Can you work these out from the model? Positions are in its coordinate system, mm. Face numbers are marked on the shaded views. A direction names the side the tool comes from. Round coordinates to 2 decimals unless told otherwise and drop trailing zeros. Order: outer loops, then holes, each group sorted by start corner. A loop starts at its lowest first (then second) coordinate and runs counter-clockwise, first axis right, second up. Notation, with made-up numbers: (49, 84) -> (62, 84) arc R14 ccw to (62, 106) -> close; hole circle Ø11 at (2.5, 27.5). An arc over 180 degrees is marked (long way). Use a Markdown table: item, result. Add a question column.
Q1. I'm going to push flat-ended pins straight in: pin 1 Ø1.4 at (x, z) = (3, 0.5) entering from -Y; pin 2 Ø2.5 at (x, z) = (8, 0.5) entering from -Y. Where does each tip first touch, or does it pass through?
Q2. If we section it at C-C on z = -2.25: List the corners of the cut face in (x, y) for me, plus the area to 3 significant figures.
Q3. If we section it at D-D on y = 6: List the corners of the cut face in (x, z) for me, plus the area to 3 significant figures.
Q4. For the marked faces 1, 2 and 3, which set-ups out of +Z, -Z, +X, -X, +Y, -Y let a thin tool reach every point of the face, with its end or its side?
Q5. We'd pull the mould along X, two halves only. Please class the marked faces 4, 5 and 6: +X half, -X half, draft (parallel to the pull), parting line (faces both ways), or undercut.
Q6. If we section it at B-B on y = 14.5: List the corners of the cut face in (x, z) for me, plus the area to 3 significant figures.
Q7. I need wall thicknesses on line 1 along Z through (x, y) = (3, 3.25); line 2 along Z through (x, y) = (5.5, 12.5); line 3 along X through (y, z) = (14.5, 0). Which ranges of each line are inside material? Lowest first, please. Write a range as [from, to].
Q8. If we section it at A-A on z = 0: List the corners of the cut face in (x, y) for me.
```python
from build123d import *

# Parameters (mm, degrees)
BOSS_EXTRUDE1_DEPTH      = 4
BOSS_EXTRUDE1_DEPTH_BACK = 4
SKETCH1_W                = 9.25
SKETCH1_H                = 17
CUT_EXTRUDE1_DEPTH       = 1.9
CUT_EXTRUDE1_DEPTH_BACK  = 1.9
SKETCH2_W                = 9.25
SKETCH2_H                = 12
SKETCH3_R                = 2.54
CUT_EXTRUDE2_DEPTH       = 21.941883869
FILLET1_R                = 0.5
CUT_EXTRUDE5_DEPTH       = 21.941884033
CUT_EXTRUDE6_REACH       = 20.488
SKETCH9_W                = 1.000000032
SKETCH9_H                = 8


# Read off the part's stored shape, not the designer's step: #10-32 Tapped Hole1
with BuildPart() as part:
    # Sketch1 → Boss-Extrude1 (new, two sides: drawn at the far end of the back side and taken through both)
    with BuildSketch(Plane.XY.offset(-BOSS_EXTRUDE1_DEPTH_BACK)):
        with Locations((4.625, 8.5)):
            Rectangle(SKETCH1_W, SKETCH1_H)
    extrude(amount=BOSS_EXTRUDE1_DEPTH + BOSS_EXTRUDE1_DEPTH_BACK)

    # Sketch2 → Cut-Extrude1 (cut, two sides: drawn at the far end of the back side and taken through both)
    with BuildSketch(Plane.XY.offset(-CUT_EXTRUDE1_DEPTH_BACK)):
        with Locations((4.625, 6)):
            Rectangle(SKETCH2_W, SKETCH2_H)
    extrude(amount=CUT_EXTRUDE1_DEPTH + CUT_EXTRUDE1_DEPTH_BACK, mode=Mode.SUBTRACT)

    # Sketch3 → Cut-Extrude2 (cut, through all)
    with BuildSketch(Plane.XY.offset(4)):
        with Locations((5.25, 5.5)):
            Circle(SKETCH3_R)
    extrude(amount=-CUT_EXTRUDE2_DEPTH, mode=Mode.SUBTRACT)

    # #10-32 Tapped Hole1 outline → #10-32 Tapped Hole1 (revolve, cut)
    with BuildSketch(Plane(origin=(5.5, 0, 0), x_dir=(1, 0, 0), z_dir=(0, 0, 1))):
        Polygon((0, 7.973018958), (1.928351252, 7.973018958), (2.019302964, 8.027668689), (2.0193, 17), (0, 17), align=None)
    revolve(axis=Axis((5.5, 0, 0), (0, 1, 0)), mode=Mode.SUBTRACT)

    # Fillet1
    fillet1_edges = [part.edges().sort_by_distance(p)[0] for p in [
        (7.716900739, 12, -1.9),
        (7.716900739, 12, 1.9),
        (2.408099261, 12, -1.9),
        (2.408099261, 12, 1.9),
    ]]
    fillet(fillet1_edges, radius=FILLET1_R)

    # Sketch7 → Cut-Extrude5 (cut, through all)
    with BuildSketch(Plane.XY.offset(4)):
        with BuildLine():
            Line((5.25, 1.5), (0, 1.5))
            Line((0, 1.5), (0, 0))
            Line((0, 0), (9.25, 0))
            Line((9.25, 0), (9.25, 5.5))
            ThreePointArc((9.25, 5.5), (8.078427125, 2.671572875), (5.25, 1.5))
        make_face()
    extrude(amount=-CUT_EXTRUDE5_DEPTH, mode=Mode.SUBTRACT)

    # Sketch9 → Cut-Extrude6 (cut, up to next)
    with BuildSketch(Plane(origin=(0, 17, 0), x_dir=(1, 0, 0), z_dir=(0, 1, 0)), mode=Mode.PRIVATE) as cut_extrude6_sk1:
        with Locations((0.500000016, 0)):
            Rectangle(SKETCH9_W, SKETCH9_H)
    cut_extrude6_tool1 = extrude(cut_extrude6_sk1.sketch, amount=-CUT_EXTRUDE6_REACH, mode=Mode.PRIVATE) & part.part
    add(cut_extrude6_tool1.solids().sort_by_distance((0.5, 17, 0))[0], mode=Mode.SUBTRACT)


solid = part.part
```
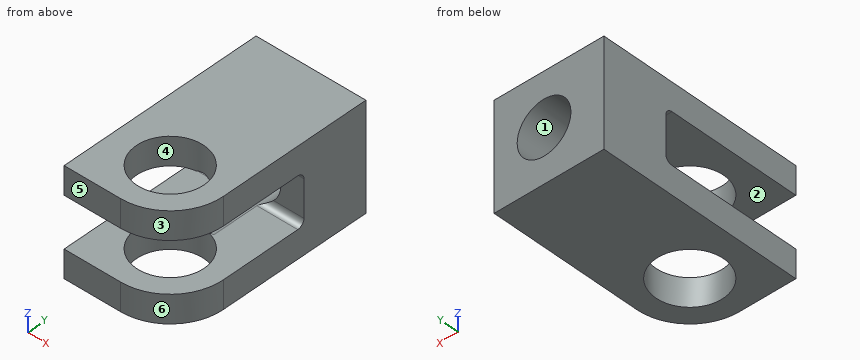
Answer below:
| question | item | result |
|---|---|---|
| 1 | pin 1 | y = 12 |
| 1 | pin 2 | y = 11.86 |
| 2 | outline | (1, 1.5) -> (5.25, 1.5) arc R4 ccw to (9.25, 5.5) -> (9.25, 17) -> (1, 17) -> close; hole circle Ø5.08 at (5.25, 5.5) |
| 2 | area | 104 mm² |
| 3 | outline | (1, -4) -> (2.76, -4) -> (2.76, -1.9) -> (1, -1.9) -> close; (1, 1.9) -> (2.76, 1.9) -> (2.76, 4) -> (1, 4) -> close; (7.74, -4) -> (9.25, -4) -> (9.25, -1.9) -> (7.74, -1.9) -> close; (7.74, 1.9) -> (9.25, 1.9) -> (9.25, 4) -> (7.74, 4) -> close |
| 3 | area | 13.7 mm² |
| 4 | face 1 | +Y |
| 4 | face 2 | +X, -X, -Y |
| 4 | face 3 | +Z, -Z, +X, -Y |
| 5 | face 4 | undercut |
| 5 | face 5 | draft |
| 5 | face 6 | +X half |
| 6 | outline | (1, -4) -> (9.25, -4) -> (9.25, 4) -> (1, 4) -> close; hole circle Ø4.04 at (5.5, 0) |
| 6 | area | 53.2 mm² |
| 7 | line 1 | [-4, -1.9], [1.9, 4] |
| 7 | line 2 | [-4, -2.02], [2.02, 4] |
| 7 | line 3 | [1, 3.48], [7.52, 9.25] |
| 8 | outline | (1, 12) -> (3.48, 12) -> (3.48, 17) -> (1, 17) -> close; (7.52, 12) -> (9.25, 12) -> (9.25, 17) -> (7.52, 17) -> close |
